```python
from build123d import *

# Parameters (mm, degrees)
F0_R     = 31.75
F1_DEPTH = 44.45
F3_DEPTH = 12.7
F4_R     = 5.08


with BuildPart() as f1:
    # F0 (on Top) → F1 (new body)
    with BuildSketch(Plane.XY):
        Circle(F0_R)
    extrude(amount=F1_DEPTH)

    # F2 (on face) → F3 (join)
    with BuildSketch(Plane.XY.offset(44.45)):
        Polygon((-16.125254, -9.30992), (16.125254, -9.30992), (0, 18.619839), align=None)
    extrude(amount=F3_DEPTH)

    # F4
    f4_edges = [f1.edges().sort_by_distance(p)[0] for p in [
        (-31.75, 0, 0),
        (-31.75, 0, 44.45),
        (0, -9.30992, 57.15),
        (-8.062627, 4.65496, 57.15),
        (8.062627, 4.65496, 57.15),
    ]]
    fillet(f4_edges, radius=F4_R)


solid = f1.part
```
Work out the finished part from the listing and answer in its coordinate system (mm). A direction names the side the tool comes from. Give positions to 0.01 mm unless a question says otherwise; leave off trailing zeros. Order: outer loops, then holes, each group sorted by start corner. A loop starts at its lowest first (then second) coordinate and runs counter-clockwise, first axis right, second up. Notation, with made-up numbers: M -25.75,33 L 22.25,33 A9 cw 22.25,48 Z; hole C -12,28.5 d10. An arc over 180 degrees is marked long. Return JSON: item names as keys, results as strings.
1) Each of these flat-tipped pins is pushed along its axis until it touches: pin 1 (3 mm diameter, centred on x = 16, z = 44, fed in from -Y); pin 2 (1 mm diameter, centred on y = 13, z = 46, fed in from +X); pin 3 (3 mm diameter, centred on y = -17.5, z = 24, fed in from +X); pin 4 (5 mm diameter, centred on x = -10, y = 1.5, fed in from -Z). Where does it stop, or does it pass through?
Resolved:
{"pin 1": "y = -26.42", "pin 2": "x = 3.53", "pin 3": "x = 27.42", "pin 4": "z = 0"}
2) Straight lines are drawn through the part: line 1 along Z through (x, y) = (12, 7.5); line 2 along Y through (x, z) = (2.5, 12.5); line 3 along X through (y, z) = (-24.5, 5). For each, find the intervals that lie inside material, in ascending order. Write a range as [from, to].
Resolved:
{"line 1": "[0, 44.45]", "line 2": "[-31.65, 31.65]", "line 3": "[-20.19, 20.19]"}
3) A tool of negligible diameter and unlimited length cuts with its end or side. For faces 1 (the flat face through (8.176, 4.459, 48.207)), 2 (the flat face through (0, 1, 57.15)), 3 (the cylindrical face through (-6.883, -30.995, 21.985)), 4 (the flat face through (-7.95, 4.85, 48.21)), 5 (the flat face through (0, -9.31, 48)), from which of +Z, -Z, +X, -X, +Y, -Y can it reach the whole face along a straight path? Write none if from no direction.
Resolved:
{"face 1": "+Z, +X, +Y", "face 2": "+Z, +X, -X, +Y, -Y", "face 3": "+Z, -Z", "face 4": "+Z, -X, +Y", "face 5": "+Z, +X, -X, -Y"}
4) Section A-A, the plane z = 16.5 is taken. Write down the section's boundary in (x, y), plus the area to 3 significant figures.
Resolved:
{"outline": "C 0,0 d63.5", "area": "3,170 mm^2"}
